For this review, take the finished solid that the model builds, in its own axes (mm). Face numbers are marked on the shaded views. A direction names the side the tool comes from. Give positions to 0.01 mm unless a question says otherwise; leave off trailing zeros. Write each loop counter-clockwise with the first axis right and the second up, starting at its lowest first coordinate (ties: lowest second). Pieces come first, ordered by that corner, then holes. Notation, with made-up numbers: M 39,31 L 43,31 A28 cw 43,68 Z; hole C 62,28 d4. An arc over 180 degrees is marked long. Use one line per item in the form item = value. Start each with the question number.
Q1. For probe 1 along X at (y, z) = (-20, 1); probe 2 along Z at (x, y) = (-71.5, 14) (3 decimals); probe 3 along X at (y, z) = (16, 0) (3 decimals), list the stretches that pass through material, from the lowest coordinate up. Write a range as [from, to].
Q2. Consider section B-B on y = -22. Write out the cut boundary in (x, z).
Q3. Tool access review of the marked faces 1 and 2: name each direction out of +Z, -Z, +X, -X, +Y, -Y from which nothing blocks a thin tool from reaching the whole face with its end or side.
Q4. Clearance check with flat-ended pins moving along their axes: pin 1 Ø10.5 at (x, y) = (-50, -1.5) entering from +Z (3 decimals); pin 2 Ø1.5 at (x, y) = (-66, -19) entering from +Z (3 decimals); pin 3 Ø0.7 at (y, z) = (0, 1) entering from +X (3 decimals); pin 4 Ø5 at (x, y) = (-18, 23) entering from -Z. State where each tip first meets the part, or that it passes through.
Q5. Consider section A-A on x = 0. Write out the cut boundary in (y, z), and give its area (3 significant figures).
```python
from build123d import *

# Parameters (mm, degrees)
F1_R          = 12.7
F2_DEPTH      = 101.6
F3_R          = 5.08
F4_W          = 38.1
F4_H          = 6.35
F5_DEPTH      = 101.6
F6_DEPTH      = 101.6
F7_W          = 2.9432778758
F7_H          = 15.875
F8_DEPTH      = 25.4
F9_W          = 2.9432778758
F9_H          = 15.875
F10_DEPTH     = 25.4
F11_W         = 1.905
F11_H         = 16.1925
F11_W_2       = 18.7325
F11_H_2       = 1.905
F11_W_3       = 44.2182778758
F11_W_4       = 1.8969494015
F11_W_5       = 18.7405505985
F12_DEPTH     = 2.54
F13_W         = 18.7325
F13_H         = 1.905
F13_W_2       = 1.9137861806
F13_H_2       = 16.1925
F13_W_3       = 44.2094916952
F13_W_4       = 1.905
F13_W_5       = 18.3292221242
F14_DEPTH     = 2.54
F15_T1_DEPTH  = 57.6962243683
F15_T3_DEPTH  = 62.7762243683
F15_T5_DEPTH  = 62.7762243683
F15_T10_DEPTH = 62.7762243683
F15_S11_R     = 12.7
F15_T12_DEPTH = 33
F15_T16_DEPTH = 62.7762243683
F15_S17_R     = 12.7
F15_T18_DEPTH = 33
F15_T22_DEPTH = 62.7762243683
F15_S23_R     = 12.7
F15_T24_DEPTH = 33
F15_T28_DEPTH = 62.7762243683
F15_S29_R     = 12.7
F15_T30_DEPTH = 33
F17_R         = 19.05
F18_DEPTH     = 19.05
F19_R         = 5.08


# Not quite as in the source:
# - a fillet or chamfer that OpenCascade refuses, or shapes differently, is made with other operations: its cross-section is extruded or revolved along the edge and cut away or added


with BuildPart() as f2:
    # F1 (on offset) → F2 (new body)
    with BuildSketch(Plane.XZ.offset(50.8)):
        Circle(F1_R)
    extrude(amount=-F2_DEPTH)

    # F3
    f3_edges = [f2.edges().sort_by_distance(p)[0] for p in [
        (-12.7, -50.8, 0),
        (-12.7, 50.8, 0),
    ]]
    fillet(f3_edges, radius=F3_R)

    # F4 (on Right) → F5 (join)
    with BuildSketch(Plane.YZ):
        Rectangle(F4_W, F4_H)
    extrude(amount=F5_DEPTH)

    # F4 (on Right) → F6 (join)
    with BuildSketch(Plane.YZ):
        Rectangle(F4_W, F4_H)
    extrude(amount=-F6_DEPTH)

    # F7 (on face) → F8 (cut)
    with BuildSketch(Plane.XY.offset(3.175)):
        with Locations((-56.9483610621, 11.1125)):
            Rectangle(F7_W, F7_H)
        with Locations((-56.9483610621, -11.1125)):
            Rectangle(F7_W, F7_H)
    extrude(amount=-F8_DEPTH, mode=Mode.SUBTRACT)

    # F9 (on face) → F10 (cut)
    with BuildSketch(Plane.XY.offset(3.175)):
        with Locations((56.9483610621, 11.1125)):
            Rectangle(F9_W, F9_H)
        with Locations((56.9483610621, -11.1125)):
            Rectangle(F9_W, F9_H)
    extrude(amount=-F10_DEPTH, mode=Mode.SUBTRACT)

    # F11 (on face) → F12 (cut)
    with BuildSketch(Plane.XY.offset(3.175)):
        with Locations((-80.01, 9.04875)):
            Rectangle(F11_W, F11_H)
        with Locations((-90.32875, 0)):
            Rectangle(F11_W_2, F11_H_2)
        with Locations((-80.01, 0)):
            Rectangle(F11_W, F11_H_2)
        with Locations((-80.01, -9.04875)):
            Rectangle(F11_W, F11_H)
        with Locations((-56.9483610621, 0)):
            Rectangle(F11_W_3, F11_H_2)
        with Locations((-33.8907474235, -9.04875)):
            Rectangle(F11_W_4, F11_H)
        with Locations((-33.8907474235, 0)):
            Rectangle(F11_W_4, F11_H_2)
        with Locations((-33.8907474235, 9.04875)):
            Rectangle(F11_W_4, F11_H)
        with Locations((-23.5719974235, 0)):
            Rectangle(F11_W_5, F11_H_2)
    extrude(amount=-F12_DEPTH, mode=Mode.SUBTRACT)

    # F13 (on face) → F14 (cut)
    with BuildSketch(Plane.XY.offset(3.175)):
        with Locations((23.5679721242, 0)):
            Rectangle(F13_W, F13_H)
        with Locations((33.8911152145, 9.04875)):
            Rectangle(F13_W_2, F13_H_2)
        with Locations((33.8911152145, 0)):
            Rectangle(F13_W_2, F13_H)
        with Locations((33.8911152145, -9.04875)):
            Rectangle(F13_W_2, F13_H_2)
        with Locations((56.9527541524, 0)):
            Rectangle(F13_W_3, F13_H)
        with Locations((80.01, 9.04875)):
            Rectangle(F13_W_4, F13_H_2)
        with Locations((80.01, 0)):
            Rectangle(F13_W_4, F13_H)
        with Locations((90.1271110621, 0)):
            Rectangle(F13_W_5, F13_H)
        with Locations((80.01, -9.04875)):
            Rectangle(F13_W_4, F13_H_2)
    extrude(amount=-F14_DEPTH, mode=Mode.SUBTRACT)

    # F15: chamfer of 3.81 on 10 edges, made by hand

    # F15_s2 → F15_t1 (cut)
    with BuildSketch(Plane.XZ.offset(-28.8481121842)):
        Polygon((-97.79, 3.175), (-101.6, -0.635), (-101.6, 3.175), align=None)
        Polygon((97.79, 3.175), (101.6, -0.635), (101.6, 3.175), align=None)
    extrude(amount=F15_T1_DEPTH, mode=Mode.SUBTRACT)

    # F15_s4 → F15_t3 (cut)
    with BuildSketch(Plane.YZ.offset(48.6218878158)):
        Polygon((15.24, 3.175), (19.05, -0.635), (19.05, 3.175), align=None)
        Polygon((-15.24, 3.175), (-19.05, -0.635), (-19.05, 3.175), align=None)
    extrude(amount=F15_T3_DEPTH, mode=Mode.SUBTRACT)

    # F15_s6 → F15_t5 (cut)
    with BuildSketch(Plane.YZ.offset(-111.3981121842)):
        Polygon((-15.24, 3.175), (-19.05, -0.635), (-19.05, 3.175), align=None)
        Polygon((15.24, 3.175), (19.05, -0.635), (19.05, 3.175), align=None)
    extrude(amount=F15_T5_DEPTH, mode=Mode.SUBTRACT)


with BuildPart() as f15_tool8:
    # F15_s9 → F15_t10 (new body)
    with BuildSketch(Plane.YZ.offset(2.4986099401)):
        Polygon((19.05, -0.635), (15.24, 3.175), (19.05, 3.175), align=None)
    extrude(amount=F15_T10_DEPTH)

    # F15_s11 → F15_t12 (cut, symmetric)
    with BuildSketch(Plane.XZ.offset(-17.1)):
        Circle(F15_S11_R)
    extrude(amount=F15_T12_DEPTH, both=True, mode=Mode.SUBTRACT)


with BuildPart() as f2_1:
    add(f2.part)

    # F15_t7: cut F15_tool8
    add(f15_tool8.part, mode=Mode.SUBTRACT)


with BuildPart() as f15_tool14:
    # F15_s15 → F15_t16 (new body)
    with BuildSketch(Plane.YZ.offset(2.4986099401)):
        Polygon((-19.05, -0.635), (-15.24, 3.175), (-19.05, 3.175), align=None)
    extrude(amount=F15_T16_DEPTH)

    # F15_s17 → F15_t18 (cut, symmetric)
    with BuildSketch(Plane.XZ.offset(17.1)):
        Circle(F15_S17_R)
    extrude(amount=F15_T18_DEPTH, both=True, mode=Mode.SUBTRACT)


with BuildPart() as f2_2:
    add(f2_1.part)

    # F15_t13: cut F15_tool14
    add(f15_tool14.part, mode=Mode.SUBTRACT)


with BuildPart() as f15_tool20:
    # F15_s21 → F15_t22 (new body)
    with BuildSketch(Plane.YZ.offset(-2.4986099401)):
        Polygon((-19.05, -0.635), (-15.24, 3.175), (-19.05, 3.175), align=None)
    extrude(amount=-F15_T22_DEPTH)

    # F15_s23 → F15_t24 (cut, symmetric)
    with BuildSketch(Plane.XZ.offset(17.1)):
        Circle(F15_S23_R)
    extrude(amount=F15_T24_DEPTH, both=True, mode=Mode.SUBTRACT)


with BuildPart() as f2_3:
    add(f2_2.part)

    # F15_t19: cut F15_tool20
    add(f15_tool20.part, mode=Mode.SUBTRACT)


with BuildPart() as f15_tool26:
    # F15_s27 → F15_t28 (new body)
    with BuildSketch(Plane.YZ.offset(-2.4986099401)):
        Polygon((19.05, -0.635), (15.24, 3.175), (19.05, 3.175), align=None)
    extrude(amount=-F15_T28_DEPTH)

    # F15_s29 → F15_t30 (cut, symmetric)
    with BuildSketch(Plane.XZ.offset(-17.1)):
        Circle(F15_S29_R)
    extrude(amount=F15_T30_DEPTH, both=True, mode=Mode.SUBTRACT)


with BuildPart() as f2_4:
    add(f2_3.part)

    # F15_t25: cut F15_tool26
    add(f15_tool26.part, mode=Mode.SUBTRACT)

    # F17 (on offset) → F18 (join)
    with BuildSketch(Plane.XZ.offset(25.4)):
        Circle(F17_R)
    extrude(amount=F18_DEPTH)

    # F19
    f19_edges = [f2_4.edges().sort_by_distance(p)[0] for p in [
        (-19.05, -44.45, 0),
        (-7.62, -50.8, 0),
    ]]
    fillet(f19_edges, radius=F19_R)


solid = f2_4.part
```
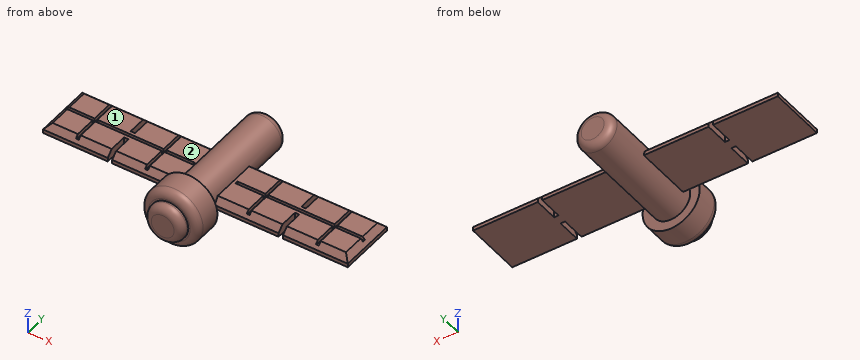
Working result:
q1.probe_1 = [-12.66, 12.66]
q1.probe_2 = [-3.175, 3.175]
q1.probe_3 = [-100.965, -58.42], [-55.477, 55.477], [58.42, 100.965]
q2.outline = C 0,0 d25.4
q3.face_1 = +Z, -X, +Y, -Y
q3.face_2 = +Z, -X, +Y
q4.pin_1 = 3.175
q4.pin_2 = 0.165
q4.pin_3 = 100.315
q4.pin_4 = through
q5.outline = M -50.8,-7.62 A5.08 ccw -45.72,-12.7 L -44.45,-12.7 L -44.45,-13.97 A5.08 ccw -39.37,-19.05 L -25.4,-19.05 L -25.4,-12.7 L 45.72,-12.7 A5.08 ccw 50.8,-7.62 L 50.8,7.62 A5.08 ccw 45.72,12.7 L -25.4,12.7 L -25.4,19.05 L -39.37,19.05 A5.08 ccw -44.45,13.97 L -44.45,12.7 L -45.72,12.7 A5.08 ccw -50.8,7.62 Z
q5.area = 2,790 mm²
